from build123d import *

# Parameters (mm, degrees)
DODANIE_WYCI_GNI_CIE1_DEPTH = 8
OTW_R_POD_RUB_M22_D         = 2.6
SKORUPA1_T                  = -3
DODANIE_WYCI_GNI_CIE2_REACH = 228.526
OTW_R_POD_RUB_M21_D         = 2.6
WYTNIJ_WYCI_GNI_CIE1_REACH  = 228.526
SZKIC7_W                    = 41
SZKIC7_H                    = 21
OTWORY_USTALAJ_CE_8_0MM1_D  = 8
OTW_R_POD_RUB_M23_D         = 2.6
WYTNIJ_WYCI_GNI_CIE2_REACH  = 228.526
SZKIC13_W                   = 5.14
SZKIC13_H                   = 8
SZKIC18_W                   = 8
SZKIC18_H                   = 6
SZKIC18_W_2                 = 6
SZKIC18_H_2                 = 4
DODANIE_WYCI_GNI_CIE3_DEPTH = 10
SZYK_LINIOWY1_COUNT         = 2
SZYK_LINIOWY1_PITCH         = 50
OTW_R_POD_RUB_M24_D         = 2.4


with BuildPart() as part:
    # Szkic1 → Dodanie-wyciągnięcie1 (new body)
    with BuildSketch(Plane.XY):
        with BuildLine():
            Line((17.853571071, 17.5), (182.146428929, 17.5))
            ThreePointArc((182.146428929, 17.5), (225, 0), (182.146428929, -17.5))
            Line((182.146428929, -17.5), (17.853571071, -17.5))
            ThreePointArc((17.853571071, -17.5), (-25, 0), (17.853571071, 17.5))
        make_face()
    extrude(amount=DODANIE_WYCI_GNI_CIE1_DEPTH)

    # Otwór pod śrubę M22 (through all)
    with Locations(Plane(origin=(0, 0, 8), x_dir=(-1, 0, 0), z_dir=(0, 0, 1))):
        with Locations((-200, 0)):
            Hole(OTW_R_POD_RUB_M22_D / 2)

    # Skorupa1
    skorupa1_openings = [part.faces().sort_by_distance(p)[0] for p in [
        (99.943079522, 0, 0),
    ]]
    offset(amount=SKORUPA1_T, openings=skorupa1_openings, kind=Kind.INTERSECTION)

    # Szkic15 → Dodanie-wyciągnięcie2 (add, up to next)
    with BuildSketch(Plane(origin=(0, 0, 0), x_dir=(-1, 0, 0), z_dir=(0, 0, -1)), mode=Mode.PRIVATE) as dodanie_wyci_gni_cie2_sk1:
        with BuildLine():
            Line((-16.545392108, -14.5), (-19.124591499, -14.5))
            ThreePointArc((-19.124591499, -14.5), (-24, 0), (-19.124591499, 14.5))
            Line((-19.124591499, 14.5), (-16.545392108, 14.5))
            ThreePointArc((-16.545392108, 14.5), (-22, 0), (-16.545392108, -14.5))
        make_face()
    dodanie_wyci_gni_cie2_tool1 = extrude(dodanie_wyci_gni_cie2_sk1.sketch, amount=-DODANIE_WYCI_GNI_CIE2_REACH, mode=Mode.PRIVATE) - part.part
    # Szkic15 → Dodanie-wyciągnięcie2 (add, up to next)
    with BuildSketch(Plane(origin=(0, 0, 0), x_dir=(-1, 0, 0), z_dir=(0, 0, -1)), mode=Mode.PRIVATE) as dodanie_wyci_gni_cie2_sk2:
        with BuildLine():
            Line((-180.875408501, -14.5), (-183.454607892, -14.5))
            ThreePointArc((-183.454607892, -14.5), (-178, 0), (-183.454607892, 14.5))
            Line((-183.454607892, 14.5), (-180.875408501, 14.5))
            ThreePointArc((-180.875408501, 14.5), (-176, 0), (-180.875408501, -14.5))
        make_face()
    dodanie_wyci_gni_cie2_tool2 = extrude(dodanie_wyci_gni_cie2_sk2.sketch, amount=-DODANIE_WYCI_GNI_CIE2_REACH, mode=Mode.PRIVATE) - part.part
    add(dodanie_wyci_gni_cie2_tool1.solids().sort_by_distance((17.834992, 14.200572, 0))[0])
    add(dodanie_wyci_gni_cie2_tool2.solids().sort_by_distance((182.165008, -14.200572, 0))[0])

    # Otwór pod śrubę M21 (through all)
    with Locations(Plane.XY.offset(8)):
        with Locations((7.1, 0), (-7.1, 0)):
            Hole(OTW_R_POD_RUB_M21_D / 2)

    # Szkic7 → Wytnij-wyciągnięcie1 (cut, up to next)
    with BuildSketch(Plane(origin=(0, 0, 0), x_dir=(-1, 0, 0), z_dir=(0, 0, -1)), mode=Mode.PRIVATE) as wytnij_wyci_gni_cie1_sk1:
        with Locations((-55, 0)):
            Rectangle(SZKIC7_W, SZKIC7_H)
    wytnij_wyci_gni_cie1_tool1 = extrude(wytnij_wyci_gni_cie1_sk1.sketch, amount=-WYTNIJ_WYCI_GNI_CIE1_REACH, mode=Mode.PRIVATE) & part.part
    add(wytnij_wyci_gni_cie1_tool1.solids().sort_by_distance((55, 0, 0))[0], mode=Mode.SUBTRACT)

    # Otwory ustalające Ø8.0mm1 (through all)
    with Locations(Plane(origin=(0, 0, 8), x_dir=(-1, 0, 0), z_dir=(0, 0, 1))):
        with Locations((0, 0)):
            Hole(OTWORY_USTALAJ_CE_8_0MM1_D / 2)

    # Otwór pod śrubę M23 (through all)
    with Locations(Plane(origin=(0, 0, 8), x_dir=(-1, 0, 0), z_dir=(0, 0, 1))):
        with Locations((-80.03, 5), (-80.03, -5), (-30.25, -5), (-30.25, 5)):
            Hole(OTW_R_POD_RUB_M23_D / 2)

    # Szkic13 → Wytnij-wyciągnięcie2 (cut, up to next)
    with BuildSketch(Plane(origin=(0, 0, 0), x_dir=(-1, 0, 0), z_dir=(0, 0, -1)), mode=Mode.PRIVATE) as wytnij_wyci_gni_cie2_sk1:
        with Locations((-75.57, 0)):
            Rectangle(SZKIC13_W, SZKIC13_H)
    wytnij_wyci_gni_cie2_tool1 = extrude(wytnij_wyci_gni_cie2_sk1.sketch, amount=-WYTNIJ_WYCI_GNI_CIE2_REACH, mode=Mode.PRIVATE) & part.part
    add(wytnij_wyci_gni_cie2_tool1.solids().sort_by_distance((75.57, 0, 0))[0], mode=Mode.SUBTRACT)

    # Szkic18 → Dodanie-wyciągnięcie3 (add)
    with BuildSketch(Plane(origin=(50, 0, 0), x_dir=(0, 0, -1), z_dir=(1, 0, 0))):
        with Locations((-4, 20.5)):
            Rectangle(SZKIC18_W, SZKIC18_H)
        with Locations((-4, 20.5)):
            Rectangle(SZKIC18_W_2, SZKIC18_H_2, mode=Mode.SUBTRACT)
    dodanie_wyci_gni_cie3 = extrude(amount=DODANIE_WYCI_GNI_CIE3_DEPTH)

    # Szyk liniowy1: Dodanie-wyciągnięcie3 ×2
    with Locations(*[(i * SZYK_LINIOWY1_PITCH, 0, 0) for i in range(1, SZYK_LINIOWY1_COUNT)]):
        add(dodanie_wyci_gni_cie3)

    # Otwór pod śrubę M24 (through all)
    with Locations(Plane(origin=(0, 0, 5), x_dir=(-1, 0, 0), z_dir=(0, 0, -1))):
        with Locations((-145, -10), (-145, 10), (-95, 10), (-95, -10)):
            Hole(OTW_R_POD_RUB_M24_D / 2)

    # Cięcie powierzchnią1
    split(bisect_by=Plane(origin=(120, 0, 0), x_dir=(0, 0, -1), z_dir=(1, 0, 0)), keep=Keep.BOTTOM)


solid = part.part
The model under review builds one solid part; all positions refer to its coordinate system, in mm. A direction names the side the tool comes from. Give positions to 0.01 mm unless a question says otherwise; leave off trailing zeros. Loops run counter-clockwise (first coordinate to the right, second up) from the corner with the lowest first, then second, coordinate; pieces in that order, holes last. Notation, with made-up numbers: (26, 14) -> (59, 14) arc R9 ccw to (59, 22) -> close; hole circle Ø10 at (4.5, 55.25). An arc over 180 degrees is marked (long way). Answer as a JSON object with one key per item and string values. Group by question number.
Q1. Take a section at A-A (x = 74). Write out the cut boundary in (y, z), plus the area to 3 significant figures.
Q2. Insertion check: pin 1 (3 mm diameter, centred on x = 95, z = 1.5, fed in from -Y); pin 2 (10.5 mm diameter, centred on x = 0, y = 0, fed in from -Z); pin 3 (1 mm diameter, centred on x = -3, z = 6, fed in from -Y). Each pin has a flat end and moves straight along its axis. Give the tip position at first contact, or say it passes through.
Q3. Tool access review of faces 4 (the flat face through (80, 17.5, 4)), 5 (the flat face through (55, 23.5, 4)), 6 (the flat face through (55, 10.5, 6)), 7 (the flat face through (70, -14.5, 2)): name each direction out of +Z, -Z, +X, -X, +Y, -Y from which nothing blocks a thin tool from reaching the whole face with its end or side.
Q4. Wall thickness on line 1 along Y through (x, z) = (80.03, 7.25); line 2 along Y through (x, z) = (95, 6.1); line 3 along Y through (x, z) = (0, 2.2): over which ranges is each line inside the solid? List them lowest first.
Q5. Take a section at C-C (x = 30.25). Write out the cut boundary in (y, z), plus the area to 3 significant figures.
Q6. Take a section at B-B (y = 0). Write out the cut boundary in (x, z), plus the area to 3 significant figures.
Q7. Take a section at D-D (y = -20). Write out the cut boundary in (x, z), plus the area to 3 significant figures.
Q8. Draft analysis for pull direction X (two halves, no side actions). For faces 1 (the flat face through (110, 23, 4)), 2 (the flat face through (105, 22.5, 4)), 3 (the flat face through (100, 23, 4)), state which applies: pulls with the +X half, pulls with the -X half, needs draft (parallel to the pull), parting line crosses it, or undercut.
Answer below:
{
 "1": {"outline": "(-17.5, 0) -> (-14.5, 0) -> (-14.5, 5) -> (-10.5, 5) -> (-10.5, 8) -> (-17.5, 8) -> close; (10.5, 5) -> (14.5, 5) -> (14.5, 0) -> (17.5, 0) -> (17.5, 8) -> (10.5, 8) -> close", "area": "72.0 mm2"},
 "2": {"pin 1": "stops at y = -17.5", "pin 2": "stops at z = 5", "pin 3": "stops at y = -24.87"},
 "3": {"face 4": "+Z, -Z, +Y", "face 5": "+Z, -Z, +X, +Y", "face 6": "+Z, -Z", "face 7": "-Z, +X"},
 "4": {"line 1": "y = -17.5 to -6.3, -3.7 to 3.7, 6.3 to 17.5", "line 2": "y = -17.5 to -11.2, -8.8 to 8.8, 11.2 to 17.5", "line 3": "y = -25 to -22, 22 to 25"},
 "5": {"outline": "(-17.5, 0) -> (-14.5, 0) -> (-14.5, 5) -> (-6.3, 5) -> (-6.3, 8) -> (-17.5, 8) -> close; (-3.7, 5) -> (3.7, 5) -> (3.7, 8) -> (-3.7, 8) -> close; (6.3, 5) -> (14.5, 5) -> (14.5, 0) -> (17.5, 0) -> (17.5, 8) -> (6.3, 8) -> close", "area": "119 mm2"},
 "6": {"outline": "(-25, 0) -> (-22, 0) -> (-22, 5) -> (-8.4, 5) -> (-8.4, 8) -> (-25, 8) -> close; (-5.8, 5) -> (-4, 5) -> (-4, 8) -> (-5.8, 8) -> close; (4, 5) -> (5.8, 5) -> (5.8, 8) -> (4, 8) -> close; (8.4, 5) -> (22, 5) -> (22, 0) -> (24, 0) -> (24, 5) -> (34.5, 5) -> (34.5, 8) -> (8.4, 8) -> close; (78.14, 5) -> (120, 5) -> (120, 8) -> (78.14, 8) -> close", "area": "289 mm2"},
 "7": {"outline": "(-15, 0) -> (-9.17, 0) -> (-9.17, 5) -> (9.17, 5) -> (9.17, 0) -> (15, 0) -> (15, 8) -> (-15, 8) -> close", "area": "148 mm2"},
 "8": {"face 1": "pulls with the +X half", "face 2": "needs draft", "face 3": "undercut"}
}
